The model under review builds one solid part; all positions refer to its coordinate system, in mm. A direction names the side the tool comes from. Coordinates: 2 decimals unless noted, no trailing zeros. Order: outer loops, then holes, each group sorted by start corner. A loop starts at its lowest first (then second) coordinate and runs counter-clockwise, first axis right, second up.
```python
from build123d import *

# Parameters (mm, degrees)
F1_DEPTH    = 15.875
F2_DEPTH    = 15.875
F3_R        = 12.7
F4_DEPTH    = 19.05
F5_R        = 2.54
F6_T1_DEPTH = 31.75
F7_R        = 0.762


# Not quite as in the source:
# - a fillet or chamfer that OpenCascade refuses, or shapes differently, is made with other operations: its cross-section is extruded or revolved along the edge and cut away or added


with BuildPart() as f1:
    # F0 (on Top) → F1 (new body, symmetric)
    with BuildSketch(Plane.XY):
        with BuildLine():
            ThreePointArc((15.875, -10.9831139027), (18.4268203443, -5.7529738397), (19.304, 0))
            ThreePointArc((19.304, 0), (18.6462321507, 4.9962428467), (16.7177543947, 9.652))
            Line((16.7177543947, 9.652), (14.518049869, 8.382))
            ThreePointArc((14.518049869, 8.382), (16.1927805519, 4.3388424721), (16.764, 0))
            ThreePointArc((16.764, 0), (-4.3388424721, -16.1927805519), (-14.518049869, 8.382))
            Line((-14.518049869, 8.382), (-16.7177543947, 9.652))
            ThreePointArc((-16.7177543947, 9.652), (-19.2879208626, -0.7877339639), (-15.875, -10.9831139027))
            ThreePointArc((-15.875, -10.9831139027), (0, -19.304), (15.875, -10.9831139027))
        make_face()
    extrude(amount=F1_DEPTH, both=True)

    # F0 (on Top) → F2 (join, symmetric)
    with BuildSketch(Plane.XY):
        with BuildLine():
            Line((15.875, -20.1168), (15.875, -10.9831139027))
            ThreePointArc((15.875, -10.9831139027), (0, -19.304), (-15.875, -10.9831139027))
            Line((-15.875, -10.9831139027), (-15.875, -20.1168))
            Line((-15.875, -20.1168), (15.875, -20.1168))
        make_face()
    extrude(amount=F2_DEPTH, both=True)

    # F3 (on face) → F4 (join)
    with BuildSketch(Plane.XZ.offset(20.1168)):
        Circle(F3_R)
    extrude(amount=F4_DEPTH)

    # F5
    f5_edges = [f1.edges().sort_by_distance(p)[0] for p in [
        (-15.875, -20.1168, 0),
        (15.875, -20.1168, 0),
        (0, -20.1168, 15.875),
        (0, -20.1168, -15.875),
    ]]
    fillet(f5_edges, radius=F5_R)

    # F6: fillet of radius 12.7 on 2 edges, made by hand

    # F6_s2 → F6_t1 (join)
    with BuildSketch(Plane.XY.offset(-15.875)):
        with BuildLine():
            ThreePointArc((-15.875, -14.4126816034), (-16.2198608148, -11.4732027866), (-17.2357142857, -8.6933635068))
            ThreePointArc((-17.2357142857, -8.6933635068), (-16.594896485, -9.8617354788), (-15.875, -10.9831139027))
            Line((-15.875, -10.9831139027), (-15.875, -14.4126816034))
        make_face()
        with BuildLine():
            ThreePointArc((15.875, -14.4126816034), (16.2198608148, -11.4732027866), (17.2357142857, -8.6933635068))
            ThreePointArc((17.2357142857, -8.6933635068), (16.594896485, -9.8617354788), (15.875, -10.9831139027))
            Line((15.875, -10.9831139027), (15.875, -14.4126816034))
        make_face()
    extrude(amount=F6_T1_DEPTH)

    # F7
    f7_edges = [f1.edges().sort_by_distance(p)[0] for p in [
        (-16.717754, 9.652, 0),
        (-14.51805, 8.382, 0),
        (16.717754, 9.652, 0),
        (14.51805, 8.382, 0),
    ]]
    fillet(f7_edges, radius=F7_R)


solid = f1.part
```
(1) Machinability: for faces 4 (the face through (-15.875, -16, 0)), 5 (the face through (-2.75, -29.51, -12.4)), 6 (the face through (16.21, -11.51, -0.22)), which of the approach directions +Z, -Z, +X, -X, +Y, -Y give a long, thin tool a straight path to every point of the face, cutting with its end or side? Answer none if there is none.
A:
face 4: +Z, -Z, -X, -Y
face 5: -Y
face 6: +Z, -Z, +X, -Y
(2) We need section B-B, the plane z = 6.5. Write out the cut boundary in (x, y) (3 decimals), and give its area (3 significant figures).
A:
outline: (-17.236, -8.693) arc R12.7 cw to (-15.875, -14.413) - (-15.875, -17.577) arc R2.54 ccw to (-13.335, -20.117) - (-10.911, -20.117) - (-10.911, -39.167) - (10.911, -39.167) - (10.911, -20.117) - (13.335, -20.117) arc R2.54 ccw to (15.875, -17.577) - (15.875, -14.413) arc R12.7 cw to (17.236, -8.693) arc R19.304 ccw to (17.1, 8.957) arc R0.762 ccw to (16.044, 9.263) - (15.164, 8.755) arc R0.762 ccw to (14.869, 7.743) arc R16.764 cw (long way) to (-14.869, 7.743) arc R0.762 ccw to (-15.164, 8.755) - (-16.044, 9.263) arc R0.762 ccw to (-17.1, 8.957) arc R19.304 ccw to start
area: 711 mm2
(3) Wall thickness on probe 1 along X at (y, z) = (0.5, -11); probe 2 along Y at (x, z) = (0, 7); probe 3 along X at (y, z) = (-12.5, 3.5): over which ranges is each line inside the solid? List them lowest first.
A:
probe 1: x = -19.3 to -16.76, 16.76 to 19.3
probe 2: y = -39.17 to -16.76
probe 3: x = -16.02 to -11.17, 11.17 to 16.02
(4) We need section C-C, the plane x = 9. Write out the cut boundary in (y, z) (3 decimals).
A:
outline: (-39.167, -8.96) - (-20.117, -8.96) - (-20.117, -13.335) arc R2.54 ccw to (-17.577, -15.875) - (-14.143, -15.875) - (-14.143, 15.875) - (-17.577, 15.875) arc R2.54 ccw to (-20.117, 13.335) - (-20.117, 8.96) - (-39.167, 8.96) - close
(5) We need section A-A, the plane y = -10. Write out the cut boundary in (x, z) (3 decimals), and give its area (3 significant figures).
A:
outline: (-16.666, -15.875) - (-13.455, -15.875) - (-13.455, 15.875) - (-16.666, 15.875) - close; (13.455, -15.875) - (16.666, -15.875) - (16.666, 15.875) - (13.455, 15.875) - close
area: 204 mm2
(6) We need section D-D, the plane y = -31. Write out the cut boundary in (x, z).
A:
outline: circle Ø25.4 at (0, 0)
(7) For pin 1 Ø6 at (x, z) = (4.5, -2.5) entering from +Y; pin 2 Ø3 at (x, y) = (8, -20.5) entering from +Z; pin 3 Ø1.6 at (y, z) = (-15.5, -3.5) entering from -X (3 decimals), all flat-tipped, find the tip position at first contact; note any pin that passes through.
A:
pin 1: stops at y = -14.99
pin 2: stops at z = 15.44
pin 3: stops at x = -15.875
(8) Draft analysis for pull direction X (two halves, no side actions). For faces 1 (the face through (0.481, -16.757, 0.222)), 2 (the face through (15.875, -16, 0)), 3 (the face through (-19.3, 0.3, 0.2)), state which applies: released by +X, released by -X, zero draft, split by the parting line, or undercut.
A:
face 1: undercut
face 2: released by +X
face 3: released by -X
